from build123d import *

# Parameters (mm, degrees)
CHAMFER1_SIZE      = 2
SKETCH7_R          = 14
CUT_EXTRUDE2_DEPTH = 41


with BuildPart() as part:
    # Sketch1 → Revolve1 (revolve)
    with BuildSketch(Plane.XY):
        Polygon((34.554515802, 18), (37.1933, 25.25), (40, 25.25), (40, 23.1186), (38.4252, 22.450137059), (38.4252, 21.187062941), (40, 20.5186), (40, 14), (40, 12), (35, 12), (35, 14), (0, 14), (0, 18), align=None)
    revolve(axis=Axis((0, 0, 0), (1, 0, 0)))

    # Chamfer1
    chamfer1_edges = [part.edges().sort_by_distance(p)[0] for p in [
        (0, -14, 0),
    ]]
    chamfer(chamfer1_edges, length=CHAMFER1_SIZE)

    # Sketch7 → Cut-Extrude2 (cut, through all)
    with BuildSketch(Plane.ZY):
        Circle(SKETCH7_R)
    extrude(amount=-CUT_EXTRUDE2_DEPTH, mode=Mode.SUBTRACT)


solid = part.part
Can you work these out from the model? Positions are in its coordinate system, mm. Round coordinates to 2 decimals unless told otherwise and drop trailing zeros. Write each loop counter-clockwise with the first axis right and the second up, starting at its lowest first coordinate (ties: lowest second). Pieces come first, ordered by that corner, then holes. Notation, with made-up numbers: M 37,72.25 L 59,72.25 A32 cw 59,103.25 Z; hole C 37.25,-10 d9. An arc over 180 degrees is marked long. Use CSV: the item, a comma, the result in double quotes.
(1) We'd pull the mould along Y, two halves only. Please class faces 1 (the cylindrical face through (17.519, -2.343, 17.847)), 2 (the flat face through (40, 4.8, -13.4)), 3 (the flat face through (38.425, 17, 13)), 4 (the conical face through (1.875, 13.473, 4.243)): +Y half, -Y half, draft (parallel to the pull), parting line (faces both ways), or undercut.
Check values:
face 1,"parting line"
face 2,"draft"
face 3,"undercut"
face 4,"undercut"
(2) I'm going to push flat-ended pins straight in: pin 1 (1 mm diameter, centred on x = 21, z = 6, fed in from -Y); pin 2 (6 mm diameter, centred on x = 32, z = 13.5, fed in from -Y); pin 3 (5 mm diameter, centred on x = 7.5, z = 12.5, fed in from +Y). Where does each tip first touch, or does it pass through?
Check values:
pin 1,"y = -17.14"
pin 2,"y = -14.62"
pin 3,"y = 14.97"
(3) Imagine slicing it at A-A (x = 17.5). Write out the boundary of the cut face in (y, z).
Check values:
outline,"C 0,0 d36; hole C 0,0 d28"
(4) I need wall thicknesses on line 1 along Z through (x, y) = (38, 0); line 2 along Z through (x, y) = (22, 12); line 3 along Y through (x, z) = (17, 5.5). Which ranges of each line are inside material? Lowest first, please.
Check values:
line 1,"-25.25 to -14, 14 to 25.25"
line 2,"-13.42 to -7.21, 7.21 to 13.42"
line 3,"-17.14 to -12.87, 12.87 to 17.14"
